Design review of the part built by this model. Coordinates are the model's own, in mm. A direction names the side the tool comes from. Coordinates: 2 decimals unless noted, no trailing zeros. Loops run counter-clockwise (first coordinate to the right, second up) from the corner with the lowest first, then second, coordinate; pieces in that order, holes last.
Q1. Wall thickness on probe 1 along Y at (x, z) = (0, 0.3); probe 2 along Y at (x, z) = (0, 1.2); probe 3 along Z at (x, y) = (-4.5, -6.5): over which ranges is each line inside the solid? List them lowest first.
Q2. Add section B-B on x = -5. Give the boundary of the cut face in (y, z) (3 decimals), and give its area (3 significant figures).
Q3. Machinability: for faces 4 (the face through (0, 13, -1)), 5 (the face through (11.084, -0.314, -0.493)), which of the approach directions +Z, -Z, +X, -X, +Y, -Y give a long, thin tool a straight path to every point of the face, cutting with its end or side? Answer none if there is none.
Q4. Draft analysis for pull direction Y (two halves, no side actions). For faces 1 (the face through (-11.084, 0.314, -0.493)), 2 (the face through (5, -6, 0.6)), 3 (the face through (6.89, -3.33, 1.5)), state which applies: released by +Y, released by -Y, zero draft, split by the parting line, or undercut.
Q5. Add section D-D on z = 1.05. Give the boundary of the cut face in (x, y), and give its area (3 significant figures).
Q6. Add section C-C on z = -0.6. Give the boundary of the cut face in (x, y), and give its area (3 significant figures).
Q7. Add section A-A on y = 0. Give the boundary of the cut face in (x, z).
Q8. For P1, Ø1, axis at x = -7, z = 0.5, coming from the +Y side; P2, Ø10, axis at x = 4.5, y = 5.5, coming from the -Z side, all flat-tipped, find the tip position at first contact; note any pin that passes through.
```python
from build123d import *

# Parameters (mm, degrees)
SCHIZZO1_R                   = 16
SCHIZZO1_R_2                 = 8
ESTRUSIONE_ESTRUSIONE1_DEPTH = 0.6
SCHIZZO3_R                   = 16
SCHIZZO3_R_2                 = 7.5
ESTRUSIONE_ESTRUSIONE2_DEPTH = 0.9
SCHIZZO5_R                   = 1.45
ESTRUSIONE_ESTRUSIONE3_DEPTH = 1
RIPETIZIONECIRCOLARE1_COUNT  = 4


with BuildPart() as part:
    # Schizzo1 → Estrusione-Estrusione1 (new body)
    with BuildSketch(Plane.XY):
        Circle(SCHIZZO1_R)
        Circle(SCHIZZO1_R_2, mode=Mode.SUBTRACT)
    extrude(amount=ESTRUSIONE_ESTRUSIONE1_DEPTH)

    # Schizzo3 → Estrusione-Estrusione2 (add)
    with BuildSketch(Plane.XY.offset(0.6)):
        Circle(SCHIZZO3_R)
        Circle(SCHIZZO3_R_2, mode=Mode.SUBTRACT)
    extrude(amount=ESTRUSIONE_ESTRUSIONE2_DEPTH)

    # Schizzo5 → Estrusione-Estrusione3 (add)
    with BuildSketch(Plane(origin=(0, 0, 0), x_dir=(-1, 0, 0), z_dir=(0, 0, -1))):
        with Locations((0, 12.5)):
            Circle(SCHIZZO5_R)
    estrusione_estrusione3 = extrude(amount=ESTRUSIONE_ESTRUSIONE3_DEPTH)

    # RipetizioneCircolare1: Estrusione-Estrusione3 ×4 about axis
    ripetizionecircolare1_axis = Axis((0, 0, 0), (0, 0, 1))
    for i in range(1, RIPETIZIONECIRCOLARE1_COUNT):
        add(estrusione_estrusione3.rotate(ripetizionecircolare1_axis, i * 360 / RIPETIZIONECIRCOLARE1_COUNT))


solid = part.part
```
Entries:
1. probe 1: y = -16 to -8, 8 to 16
1. probe 2: y = -16 to -7.5, 7.5 to 16
1. probe 3: z = 0.6 to 1.5
2. outline: (-15.199, 0) - (-6.245, 0) - (-6.245, 0.6) - (-5.59, 0.6) - (-5.59, 1.5) - (-15.199, 1.5) - close; (5.59, 0.6) - (6.245, 0.6) - (6.245, 0) - (15.199, 0) - (15.199, 1.5) - (5.59, 1.5) - close
2. area: 28.0 mm2
3. face 4: -Z, +X, -X, +Y, -Y
3. face 5: -Z
4. face 1: split by the parting line
4. face 2: undercut
4. face 3: zero draft
5. outline: circle Ø32 at (0, 0); hole circle Ø15 at (0, 0)
5. area: 628 mm2
6. outline: circle Ø2.9 at (-12.5, 0); circle Ø2.9 at (0, -12.5); circle Ø2.9 at (0, 12.5); circle Ø2.9 at (12.5, 0)
6. area: 26.4 mm2
7. outline: (-16, 0) - (-13.95, 0) - (-13.95, -1) - (-11.05, -1) - (-11.05, 0) - (-8, 0) - (-8, 0.6) - (-7.5, 0.6) - (-7.5, 1.5) - (-16, 1.5) - close; (7.5, 0.6) - (8, 0.6) - (8, 0) - (11.05, 0) - (11.05, -1) - (13.95, -1) - (13.95, 0) - (16, 0) - (16, 1.5) - (7.5, 1.5) - close
8. P1: stops at y = 14.62
8. P2: stops at z = 0
